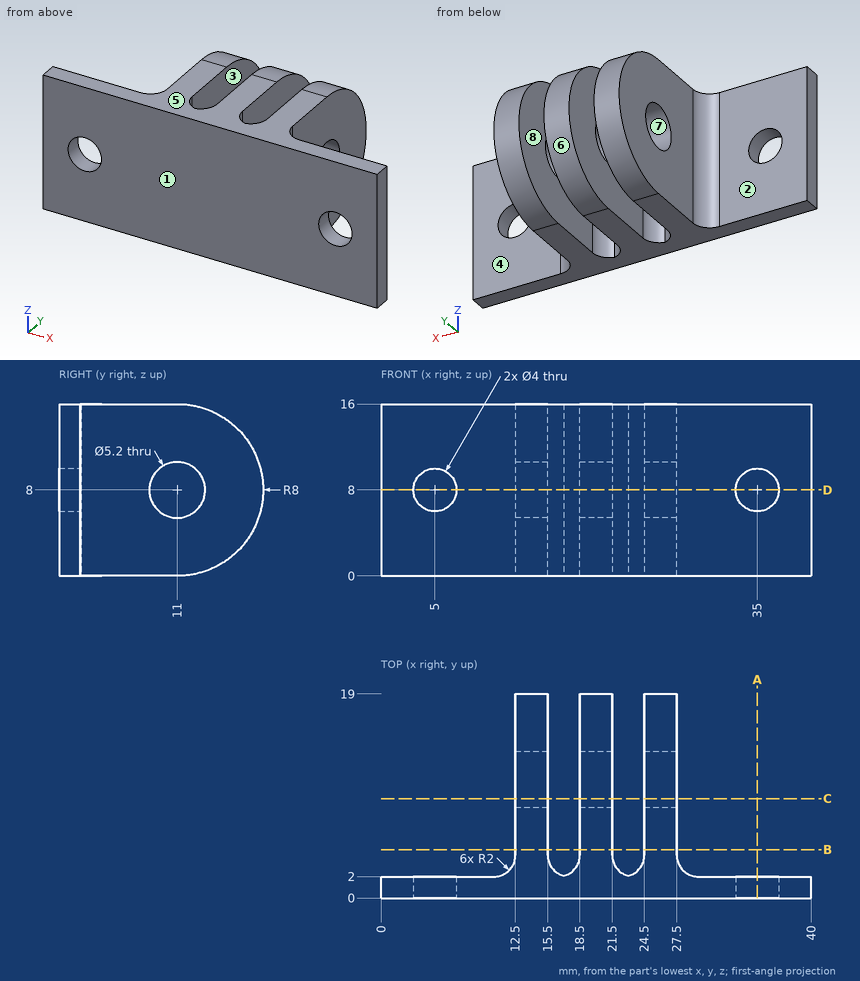
Part print with two shaded views. Sizes in mm from the minimum x, y, z corner. A direction names the side the tool comes from. Coordinates: 2 decimals unless noted, no trailing zeros. Order: outer loops, then holes, each group sorted by start corner. A loop starts at its lowest first (then second) coordinate and runs counter-clockwise, first axis right, second up.
(1) Mould opens along Z. For the marked faces 5, 6, 7 and 8 say: released by +Z, released by -Z, zero draft, split by the parting line, or undercut.
Solution:
face 5: released by +Z
face 6: split by the parting line
face 7: undercut
face 8: zero draft
(2) Saw through at B-B, the plane y = 4.5. Write the cut outline in (x, z).
Solution:
outline: (12.5, 0) - (15.5, 0) - (15.5, 16) - (12.5, 16) - close; (18.5, 0) - (21.5, 0) - (21.5, 16) - (18.5, 16) - close; (24.5, 0) - (27.5, 0) - (27.5, 16) - (24.5, 16) - close
(3) Saw through at D-D, the plane z = 8. Count the separate pieces of the cut face and the enclosed holes in it, and give its area (3 significant figures).
Solution:
separate pieces: 6
enclosed holes: 0
area: 175 mm2
(4) Drill centre lines: L1, parallel to X at y = 7.5, z = 13.5; L2, parallel to X at y = 0.9, z = 8; L3, parallel to Y at x = 14.4, z = 8. Where is each one in solid material? Low to high.
Solution:
L1: x = 12.5 to 15.5, 18.5 to 21.5, 24.5 to 27.5
L2: x = 0 to 3, 7 to 33, 37 to 40
L3: y = 0 to 8.4, 13.6 to 19
(5) Saw through at C-C, the plane y = 9.25. Write the cut outline in (x, z).
Solution:
outline: (12.5, 0) - (15.5, 0) - (15.5, 6.08) - (12.5, 6.08) - close; (12.5, 9.92) - (15.5, 9.92) - (15.5, 16) - (12.5, 16) - close; (18.5, 0) - (21.5, 0) - (21.5, 6.08) - (18.5, 6.08) - close; (18.5, 9.92) - (21.5, 9.92) - (21.5, 16) - (18.5, 16) - close; (24.5, 0) - (27.5, 0) - (27.5, 6.08) - (24.5, 6.08) - close; (24.5, 9.92) - (27.5, 9.92) - (27.5, 16) - (24.5, 16) - close
(6) Pin check, flat tips, straight feed: pin 1 Ø5 at (x, y) = (22, 12) entering from +Z; pin 2 Ø3 at (y, z) = (11, 8) entering from +X; pin 3 Ø3 at (x, z) = (3.5, 5) entering from +Y; pin 4 Ø7.5 at (y, z) = (14.5, 4) entering from -X. Stop position of each tip, or through.
Solution:
pin 1: stops at z = 16
pin 2: passes through
pin 3: stops at y = 2
pin 4: stops at x = 12.5
(7) Which spindle directions (+Z, -Z, +X, -X, +Y, -Y) get a long thin tool onto all of the face, cutting with end or side? Do the marked faces 1, 2, 3 and 4. Say none if no direction does.
Solution:
face 1: +Z, -Z, +X, -X, -Y
face 2: +Z, -Z, -X, +Y
face 3: +Z, -Z, +Y
face 4: +Z, -Z, +X, +Y
(8) Saw through at A-A, the plane x = 35. Write the cut outline in (y, z), and give its area (3 significant figures).
Solution:
outline: (0, 0) - (2, 0) - (2, 6) - (0, 6) - close; (0, 10) - (2, 10) - (2, 16) - (0, 16) - close
area: 24.0 mm2
